Read the model definition and answer for the solid it produces. Units are mm, in the model's axes. Give positions to 0.01 mm unless a question says otherwise; leave off trailing zeros.
(1) This flat-tipped pin is pushed along its axis until it touches: P1, Ø3, axis at x = 106, y = 55, coming from the -Z side. Where does it stop, or does it pass through?
(2) Determine the mould class of faces 1 (the face through (69.606, 41.621, 12.878)), 2 (the face through (333.375, 38, 13)), 3 (the face through (164, 0, 13)) for opening direction Y: pulls with the +Y half, pulls with the -Y half, needs draft (parallel to the pull), parting line crosses it, or undercut.
(3) Find section A-A, the plane y = 38.1. State how many separate pieces and enclosed holes the cut face has, then the cut area to 3 significant figures.
(4) Straight lines are drawn through the part: probe 1 along Y at (x, z) = (221.5, 11.25); probe 2 along Y at (x, z) = (76.5, 24); probe 3 along Y at (x, z) = (111, 24). For each, find the intervals that lie inside material, in ascending order.
```python
from build123d import *

# Parameters (mm, degrees)
F0_W     = 333.375
F0_H     = 76.2
F1_DEPTH = 25.4
F2_D     = 7.9375
F2_DEPTH = 50.8
F2_TIP   = 2.3846655818
F3_D     = 4.7625
F3_DEPTH = 25.4
F3_TIP   = 1.4307993491
F5_D     = 4.7625
F5_DEPTH = 25.4
F5_TIP   = 1.4307993491


# Not quite as in the source:
# - a feature names something its author has since deleted; it is built from what else it names


with BuildPart() as f1:
    # F0 (on Top) → F1 (new body)
    with BuildSketch(Plane.XY):
        with Locations((166.6875, 38.1)):
            Rectangle(F0_W, F0_H)
    extrude(amount=F1_DEPTH)

    # F2
    with Locations(Plane(origin=(0, 0, 0), x_dir=(1, 0, 0), z_dir=(0, 0, -1))):
        with Locations((15.382875, -38.1), (71.4375, -38.1), (119.0625, -38.1), (166.6875, -38.1), (214.3125, -38.1), (261.9375, -38.1), (317.992125, -38.1)):
            Hole(F2_D / 2, depth=F2_DEPTH)
            with Locations((0, 0, -(F2_DEPTH + F2_TIP / 2))):  # 118° drill point
                Cone(0, F2_D / 2, F2_TIP, mode=Mode.SUBTRACT)

    # F3
    with Locations(Plane(origin=(0, 0, 0), x_dir=(1, 0, 0), z_dir=(0, 0, -1))):
        with Locations((30.76575, -16.51), (64.48425, -16.51), (78.39075, -16.51), (112.10925, -16.51), (126.01575, -16.51), (30.76575, -59.69), (64.48425, -59.69), (78.39075, -59.69), (112.10925, -59.69), (126.01575, -59.69), (159.73425, -59.69), (173.64075, -59.69), (159.73425, -16.51), (173.64075, -16.51), (207.35925, -16.51), (221.26575, -16.51), (254.98425, -16.51), (268.89075, -16.51), (302.60925, -16.51), (207.35925, -59.69), (221.26575, -59.69), (254.98425, -59.69), (268.89075, -59.69), (302.60925, -59.69)):
            Hole(F3_D / 2, depth=F3_DEPTH)
            with Locations((0, 0, -(F3_DEPTH + F3_TIP / 2))):  # 118° drill point
                Cone(0, F3_D / 2, F3_TIP, mode=Mode.SUBTRACT)

    # F5
    with Locations(Plane.XY.offset(25.4)):
        with Locations((32.67075, 69.85), (35.02025, 49.53), (62.57925, 69.85), (60.22975, 49.53), (80.29575, 69.85), (82.64525, 49.53), (110.20425, 69.85), (107.85475, 49.53), (127.92075, 69.85), (130.27025, 49.53), (157.82925, 69.85), (155.47975, 49.53), (175.54575, 69.85), (177.89525, 49.53), (205.45425, 69.85), (203.10475, 49.53), (223.17075, 69.85), (225.52025, 49.53), (253.07925, 69.85), (250.72975, 49.53), (270.79575, 69.85), (273.14525, 49.53), (300.70425, 69.85), (298.35475, 49.53), (32.67075, 26.67), (35.02025, 6.35), (62.57925, 26.67), (60.22975, 6.35), (80.29575, 26.67), (82.64525, 6.35), (110.20425, 26.67), (107.85475, 6.35), (127.92075, 26.67), (130.27025, 6.35), (157.82925, 26.67), (155.47975, 6.35), (175.54575, 26.67), (177.89525, 6.35), (205.45425, 26.67), (203.10475, 6.35), (223.17075, 26.67), (225.52025, 6.35), (253.07925, 26.67), (250.72975, 6.35), (270.79575, 26.67), (273.14525, 6.35), (300.70425, 26.67), (298.35475, 6.35)):
            Hole(F5_D / 2, depth=F5_DEPTH)
            with Locations((0, 0, -(F5_DEPTH + F5_TIP / 2))):  # 118° drill point
                Cone(0, F5_D / 2, F5_TIP, mode=Mode.SUBTRACT)


solid = f1.part
```
Entries:
1. P1: stops at z = 0
2. face 1: undercut
2. face 2: needs draft
2. face 3: pulls with the -Y half
3. separate pieces: 8
3. enclosed holes: 0
3. area: 7,060 mm2
4. probe 1: y = 0 to 14.14, 18.88 to 24.97, 28.37 to 57.32, 62.06 to 68.15, 71.55 to 76.2
4. probe 2: y = 0 to 15.06, 17.96 to 58.24, 61.14 to 76.2
4. probe 3: y = 0 to 14.4, 18.62 to 24.43, 28.91 to 57.58, 61.8 to 67.61, 72.09 to 76.2
